```python
from build123d import *

# Parameters (mm, degrees)
F0_R     = 76.2
F1_DEPTH = 30.7
F3_D     = 25
F6_DEPTH = 50
F7_R     = 15


with BuildPart() as f1:
    # F0 (on Front) → F1 (new body)
    with BuildSketch(Plane.XZ):
        Circle(F0_R)
    extrude(amount=F1_DEPTH)

    # F3 (through all)
    with Locations(Plane.XZ.offset(30.7)):
        with Locations((0, 0)):
            Hole(F3_D / 2)

    # F5 (on face) → F6 (cut)
    with BuildSketch(Plane.XZ.offset(30.7)):
        with BuildLine():
            ThreePointArc((-17.6316000516, -5.1361640309), (-16.0992403752, 8.8356075441), (-5.1361640309, 17.6316000516))
            Line((-5.1361640309, 17.6316000516), (-15.6149722896, 53.6036124568))
            ThreePointArc((-15.6149722896, 53.6036124568), (-48.9449306583, 26.8620250703), (-53.6036124568, -15.6149722896))
            Line((-53.6036124568, -15.6149722896), (-17.6316000516, -5.1361640309))
        make_face()
        with BuildLine():
            Line((15.3924620258, 53.6679302825), (5.0629747103, 17.6527558306))
            ThreePointArc((5.0629747103, 17.6527558306), (14.6668386689, 11.0515765751), (18.3644630015, 0))
            ThreePointArc((18.3644630015, 0), (18.2675422338, -1.8842510628), (17.9778029541, -3.7486133808))
            Line((17.9778029541, -3.7486133808), (54.6561389523, -11.3965390732))
            ThreePointArc((54.6561389523, -11.3965390732), (55.5370046719, -5.7285024301), (55.8316633105, 0))
            ThreePointArc((55.8316633105, 0), (44.590141205, 33.5990168805), (15.3924620258, 53.6679302825))
        make_face()
        with BuildLine():
            Line((36.2787310037, -42.438523829), (11.9330031339, -13.9591166461))
            ThreePointArc((11.9330031339, -13.9591166461), (0.6312267901, -18.3536114722), (-10.9457629494, -14.7459748673))
            Line((-10.9457629494, -14.7459748673), (-33.277322164, -44.8307311742))
            ThreePointArc((-33.277322164, -44.8307311742), (1.9190564742, -55.7986724777), (36.2787310037, -42.438523829))
        make_face()
    extrude(amount=-F6_DEPTH, mode=Mode.SUBTRACT)

    # F7
    f7_edges = [f1.edges().sort_by_distance(p)[0] for p in [
        (-76.2, -30.7, 0),
        (76.2, -15.35, 0),
        (-76.2, 0, 0),
    ]]
    fillet(f7_edges, radius=F7_R)


solid = f1.part
```
The listing builds one solid part. Answer for the finished solid, in the listing's coordinates (mm). A direction names the side the tool comes from. Give positions to 0.01 mm unless a question says otherwise; leave off trailing zeros. Write each loop counter-clockwise with the first axis right and the second up, starting at its lowest first coordinate (ties: lowest second). Pieces come first, ordered by that corner, then holes. Notation, with made-up numbers: (-38, 87) -> (-27, 87) arc R15 cw to (-27, 93) -> close; hole circle Ø8 at (83.25, 14). An arc over 180 degrees is marked (long way). Write item = value, one per line. Start each with the question number.
1) The part is cut by section B-B, the plane y = -8.5. Determine the outline of the cut face in (x, z), and give its area (3 significant figures).
2) The part is cut by section C-C, the plane z = 30. Count the separate pieces of the cut face and the enclosed holes in it, and give its area (3 significant figures).
3) The part is cut by section A-A, the plane x = 0. Determine the outline of the cut face in (y, z).
4) Which of the six approach directions +Z, -Z, +X, -X, +Y, -Y give full straight-line access (tool end or side, diameter ignored) to faces 4 (the face through (1.393, -15.565, -55.814)), 5 (the face through (-1, 0, -13))?
5) Each of these flat-tipped pins is pushed along its axis until it touches: pin 1 (8 mm diameter, centred on y = -23.5, z = -14.5, fed in from -X); pin 2 (6 mm diameter, centred on x = -10, y = -16, fed in from -Z); pin 3 (3 mm diameter, centred on x = -44, y = -18.5, fed in from +Z). Where does it stop, or does it pass through?
6) Straight lines are drawn through the part: line 1 along Z through (x, y) = (0, -5.5); line 2 along X through (y, z) = (-13, 4.5); line 3 along Z through (x, y) = (-2.5, -11). For each, find the intervals that lie inside material, in ascending order.
7) Determine the mould class of faces 1 (the face through (-60.47, -15.345, -46.367)), 2 (the face through (-1, -30.7, -13)), 3 (the face through (0.804, -15.565, -18.347)) for opening direction Z: +Z half, -Z half, draft (parallel to the pull), parting line (faces both ways), or undercut.
8) The part is cut by section D-D, the plane y = -21. Determine the outline of the cut face in (x, z), and give its area (3 significant figures).
Solutions:
q1.outline = circle Ø149.44 at (0, 0); hole (-53.6, -15.61) -> (-17.63, -5.14) arc R18.36 cw to (-5.14, 17.63) -> (-15.61, 53.6) arc R55.83 ccw to start; hole (-33.28, -44.83) arc R55.83 ccw to (36.28, -42.44) -> (11.93, -13.96) arc R18.36 cw to (-10.95, -14.75) -> close; hole circle Ø25 at (0, 0); hole (5.06, 17.65) arc R18.36 cw to (17.98, -3.75) -> (54.66, -11.4) arc R55.83 ccw to (15.39, 53.67) -> close
q1.area = 10,900 mm²
q2.separate_pieces = 3
q2.enclosed_holes = 0
q2.area = 1,730 mm²
q3.outline = (-30.7, -61.2) arc R15 ccw to (-15.7, -76.2) -> (-15, -76.2) arc R15 ccw to (0, -61.2) -> (0, -55.83) -> (-30.7, -55.83) -> close; (-30.7, -18.36) -> (0, -18.36) -> (0, -12.5) -> (-30.7, -12.5) -> close; (-30.7, 12.5) -> (0, 12.5) -> (0, 61.2) arc R15 ccw to (-15, 76.2) -> (-15.7, 76.2) arc R15 ccw to (-30.7, 61.2) -> close
q4.face_4 = +Y, -Y
q4.face_5 = +Z, -Z, +X, -X, +Y
q5.pin_1 = -74.52
q5.pin_2 = -75.88
q5.pin_3 = 62.98
q6.line_1 = -72.81 to -55.83, -18.36 to -12.5, 12.5 to 72.81
q6.line_2 = -75.93 to -55.65, -17.8 to -11.66, 11.66 to 17.8, 55.65 to 75.93
q6.line_3 = -75.62 to -55.78, -18.19 to -12.25, 12.25 to 75.62
q7.face_1 = parting line
q7.face_2 = draft
q7.face_3 = undercut
q8.outline = circle Ø150.46 at (0, 0); hole (-53.6, -15.61) -> (-17.63, -5.14) arc R18.36 cw to (-5.14, 17.63) -> (-15.61, 53.6) arc R55.83 ccw to start; hole (-33.28, -44.83) arc R55.83 ccw to (36.28, -42.44) -> (11.93, -13.96) arc R18.36 cw to (-10.95, -14.75) -> close; hole circle Ø25 at (0, 0); hole (5.06, 17.65) arc R18.36 cw to (17.98, -3.75) -> (54.66, -11.4) arc R55.83 ccw to (15.39, 53.67) -> close
q8.area = 11,200 mm²
